Here's how the part is built. I have some questions about the finished solid (model axes, mm). A direction names the side the tool comes from. Coordinates: 2 decimals unless noted, no trailing zeros. Write each loop counter-clockwise with the first axis right and the second up, starting at its lowest first coordinate (ties: lowest second). Pieces come first, ordered by that corner, then holes.
Item 1: If I drill on line 1 (Z direction, x = 11, y = 57.5); line 2 (Z direction, x = 71, y = 15); line 3 (Y direction, x = 119, z = 22), over which ranges is the centre line in solid material (lowest first)?
Item 2: We'd pull the mould along Z, two halves only. Please class faces 1 (the face through (69, 49, 15)), 2 (the face through (69, 30, 25)), 3 (the face through (92.5, 39.84, -20.07)): +Z half, -Z half, draft (parallel to the pull), parting line (faces both ways), or undercut.
Item 3: If we section it at C-C (z = 0): Please give me the cut outline in (x, y).
Item 4: If we section it at D-D (y = 15): Please give me the cut outline in (x, z).
Item 5: I'm going to push flat-ended pins straight in: pin 1 Ø5 at (x, z) = (129, -43.5) entering from +Y; pin 2 Ø24 at (x, y) = (43.5, 39) entering from -Z; pin 3 Ø8 at (x, z) = (120, -44.5) entering from -Y. Where does each tip first touch, or does it pass through?
Item 6: For faces 4 (the face through (69, 48, -15)), 5 (the face through (125, 18.85, -44)), 6 (the face through (50, 32.5, -20)), 7 (the face through (126, 46.65, -44)), which set-ups out of +Z, -Z, +X, -X, +Y, -Y let a thin tool reach every point of the face, with its end or its side?
Item 7: If we section it at A-A (x = 89.5): Please give me the cut outline in (y, z).
Item 8: If we section it at B-B (y = 40): Please give me the cut outline in (x, z), then the cut area to 3 significant figures.
from build123d import *

# Parameters (mm, degrees)
BOSS_EXTRUDE1_DEPTH     = 139
SKETCH3_R               = 7.5
CUT_EXTRUDE1_DEPTH      = 160.439643753
CUT_EXTRUDE2_DEPTH      = 154.447059275
CUT_EXTRUDE2_DEPTH_BACK = 154.447059275
SKETCH4_R               = 7.5
SKETCH5_W               = 30
SKETCH5_H               = 60
BOSS_EXTRUDE2_DEPTH     = 13.7
SKETCH6_W               = 27.582278357
SKETCH6_H               = 4.25
SKETCH6_W_2             = 27.382278357
BOSS_EXTRUDE3_DEPTH     = 10
CUT_EXTRUDE3_DEPTH      = 136.757894005
CUT_EXTRUDE3_DEPTH_BACK = 136.757894005
SKETCH7_R               = 1


with BuildPart() as part:
    # Sketch2 → Boss-Extrude1 (new body)
    with BuildSketch(Plane(origin=(0, 0, 0), x_dir=(0, 0, -1), z_dir=(1, 0, 0))):
        Polygon((-15, 30), (15, 30), (15, 60), (25, 60), (25, 51.134717436), (25, 0), (-25, 0), (-25, 60), (-15, 60), align=None)
    extrude(amount=BOSS_EXTRUDE1_DEPTH)

    # Sketch3 → Cut-Extrude1 (cut, through all)
    with BuildSketch(Plane(origin=(0, 0, -25), x_dir=(-1, 0, 0), z_dir=(0, 0, -1))):
        with Locations((-119, 40)):
            Circle(SKETCH3_R)
        with BuildLine():
            Line((-85, 47.5), (-15, 47.5))
            ThreePointArc((-15, 47.5), (-7.5, 40), (-15, 32.5))
            Line((-15, 32.5), (-85, 32.5))
            ThreePointArc((-85, 32.5), (-92.5, 40), (-85, 47.5))
        make_face()
    extrude(amount=-CUT_EXTRUDE1_DEPTH, mode=Mode.SUBTRACT)

    # Sketch4 → Cut-Extrude2 (cut, two sides: drawn at the far end of the back side and taken through both)
    with BuildSketch(Plane(origin=(139, 0, 0), x_dir=(0, 0, -1), z_dir=(1, 0, 0)).offset(-CUT_EXTRUDE2_DEPTH_BACK)):
        with Locations((0, 15)):
            Circle(SKETCH4_R)
    extrude(amount=CUT_EXTRUDE2_DEPTH + CUT_EXTRUDE2_DEPTH_BACK, mode=Mode.SUBTRACT)

    # Sketch5 → Boss-Extrude2 (add)
    with BuildSketch(Plane(origin=(0, 0, -25), x_dir=(-1, 0, 0), z_dir=(0, 0, -1))):
        with Locations((-124, 30)):
            Rectangle(SKETCH5_W, SKETCH5_H)
    extrude(amount=BOSS_EXTRUDE2_DEPTH)

    # Sketch6 → Boss-Extrude3 (add)
    with BuildSketch(Plane(origin=(0, 0, -38.7), x_dir=(-1, 0, 0), z_dir=(0, 0, -1))):
        with Locations((-125.208860821, 20.975)):
            Rectangle(SKETCH6_W, SKETCH6_H)
        with Locations((-125.308860822, 48.775)):
            Rectangle(SKETCH6_W_2, SKETCH6_H)
    extrude(amount=BOSS_EXTRUDE3_DEPTH)

    # Sketch7 → Cut-Extrude3 (cut, two sides: drawn at the far end of the back side and taken through both)
    with BuildSketch(Plane.ZY.offset(-111.617721643).offset(-CUT_EXTRUDE3_DEPTH_BACK)):
        with Locations((-45.013158899, 48.529439721)):
            Circle(SKETCH7_R)
        with Locations((-45.013158899, 21.190661747)):
            Circle(SKETCH7_R)
    extrude(amount=CUT_EXTRUDE3_DEPTH + CUT_EXTRUDE3_DEPTH_BACK, mode=Mode.SUBTRACT)


solid = part.part
Answer list:
1. line 1: z = -25 to -15, 15 to 25
1. line 2: z = -25 to -7.5, 7.5 to 25
1. line 3: y = 0 to 32.5, 47.5 to 60
2. face 1: undercut
2. face 2: +Z half
2. face 3: draft
3. outline: (0, 0) - (139, 0) - (139, 7.5) - (0, 7.5) - close; (0, 22.5) - (139, 22.5) - (139, 30) - (0, 30) - close
4. outline: (0, -25) - (109, -25) - (109, -38.7) - (139, -38.7) - (139, -7.5) - (0, -7.5) - close; (0, 7.5) - (139, 7.5) - (139, 25) - (0, 25) - close
5. pin 1: stops at y = 50.9
5. pin 2: stops at z = -25
5. pin 3: stops at y = 18.85
6. face 4: +X, -X, +Y
6. face 5: -Z, +X, -X, -Y
6. face 6: +Z, -Z
6. face 7: -Z, +X, -X
7. outline: (0, -25) - (34, -25) - (34, -15) - (30, -15) - (30, 15) - (34, 15) - (34, 25) - (0, 25) - close; (46, -25) - (60, -25) - (60, -15) - (46, -15) - close; (46, 15) - (60, 15) - (60, 25) - (46, 25) - close; hole circle Ø15 at (15, 0)
8. outline: (0, -25) - (7.5, -25) - (7.5, -15) - (0, -15) - close; (0, 15) - (7.5, 15) - (7.5, 25) - (0, 25) - close; (92.5, -25) - (109, -25) - (109, -38.7) - (139, -38.7) - (139, -15) - (126.5, -15) - (126.5, -25) - (111.5, -25) - (111.5, -15) - (92.5, -15) - close; (92.5, 15) - (111.5, 15) - (111.5, 25) - (92.5, 25) - close; (126.5, 15) - (139, 15) - (139, 25) - (126.5, 25) - close
8. area: 1,190 mm2
